Could you check a few things on this model? Use its own coordinates, in mm. Coordinates: 2 decimals unless noted, no trailing zeros. Write each loop counter-clockwise with the first axis right and the second up, starting at its lowest first coordinate (ties: lowest second). Pieces come first, ordered by that corner, then holes.
```python
from build123d import *

# Parameters (mm, degrees)
CROQUIS1_R              = 4.05
SALIENTE_EXTRUIR1_DEPTH = 5
REDONDEO6_R             = 4


with BuildPart() as part:
    # Croquis1 → Saliente-Extruir1 (new, symmetric)
    with BuildSketch(Plane(origin=(0, 0, 0), x_dir=(-1, 0, 0), z_dir=(0, 1, 0))):
        with BuildLine():
            Line((0, -7.5), (250, -7.5))
            ThreePointArc((250, -7.5), (257.5, 0), (250, 7.5))
            Line((250, 7.5), (0, 7.5))
            ThreePointArc((0, 7.5), (-7.5, 0), (0, -7.5))
        make_face()
        with Locations(Location((0, 0, 0), (0, 0, 90))):
            Circle(CROQUIS1_R, mode=Mode.SUBTRACT)
        with Locations(Location((250, 0, 0), (0, 0, 90))):
            Circle(CROQUIS1_R, mode=Mode.SUBTRACT)
    extrude(amount=SALIENTE_EXTRUIR1_DEPTH, both=True)

    # Redondeo6
    redondeo6_edges = [part.edges().sort_by_distance(p)[0] for p in [
        (-125, 5, 7.5),
        (-125, -5, 7.5),
        (-125, 5, -7.5),
        (-125, -5, -7.5),
    ]]
    fillet(redondeo6_edges, radius=REDONDEO6_R)


solid = part.part
```
1. If we mould it in two halves opening along Z, with no side actions, what happens to faces 1 (the face through (-3.593, -0.07, 1.869)), 2 (the face through (-123.279, -3.797, 6.359)), 3 (the face through (-126.721, 3.797, -6.359))? For each: pulls with the +Z half, pulls with the -Z half, needs draft (parallel to the pull), parting line crosses it, or undercut.
Verdict:
face 1: undercut
face 2: pulls with the +Z half
face 3: pulls with the -Z half
2. I want a section at B-B on z = 0. Give the number of separate pieces and of enclosed holes in the cut face, plus the area to 3 significant figures.
Verdict:
separate pieces: 3
enclosed holes: 0
area: 2,470 mm2
3. Please list where these lines run through material, in increasing order: line 1 along X through (y, z) = (0.75, -0.25); line 2 along X through (y, z) = (0.25, -2.5); line 3 along Z through (x, y) = (-250, -1.5).
Verdict:
line 1: x = -257.5 to -254.04, -245.96 to -4.04, 4.04 to 7.5
line 2: x = -257.07 to -253.19, -246.81 to -3.19, 3.19 to 7.07
line 3: z = -7.47 to -4.05, 4.05 to 7.47
4. I want a section at A-A on x = -87. Please give me the cut outline in (y, z), plus the area to 3 significant figures.
Verdict:
outline: (-5, -3.5) arc R4 ccw to (-1, -7.5) - (1, -7.5) arc R4 ccw to (5, -3.5) - (5, 3.5) arc R4 ccw to (1, 7.5) - (-1, 7.5) arc R4 ccw to (-5, 3.5) - close
area: 136 mm2
5. For pin 1 (6.5 mm diameter, centred on x = 0, z = 0, fed in from +Y); pin 2 (1.5 mm diameter, centred on x = -62, z = 6, fed in from -Y); pin 3 (3 mm diameter, centred on y = 1.5, z = 5.5, fed in from -X); pin 4 (5 mm diameter, centred on y = 0.5, z = -3, fed in from +X), each with a flat end and sliding along its axis, tell me the tip position at first contact or that it passes through.
Verdict:
pin 1: passes through
pin 2: stops at y = -4.6
pin 3: stops at x = -256.33
pin 4: stops at x = 7.48
